```python
from build123d import *

# Parameters (mm, degrees)
BOSS_EXTRUDE1_DEPTH = 30
SKETCH2_R           = 2
CUT_EXTRUDE1_DEPTH  = 3
FILLET1_R           = 3


with BuildPart() as part:
    # Sketch1 → Boss-Extrude1 (new body)
    with BuildSketch(Plane(origin=(-298.953701388, 67.353578403, 0), x_dir=(1, 0, 0), z_dir=(0, 0, 1))):
        Polygon((318.453701388, -54.353578403), (318.453701388, -64.353578403), (313.453701388, -64.353578403), (313.453701388, -54.353578403), (310.453701388, -54.353578403), (310.453701388, -64.353578403), (298.953701388, -64.353578403), (298.953701388, -67.353578403), (332.953701388, -67.353578403), (332.953701388, -64.353578403), (321.453701388, -64.353578403), (321.453701388, -54.353578403), align=None)
    extrude(amount=BOSS_EXTRUDE1_DEPTH)

    # Sketch2 → Cut-Extrude1 (cut)
    with BuildSketch(Plane(origin=(0, 3, 0), x_dir=(1, 0, 0), z_dir=(0, 1, 0))):
        with Locations(Location((29, -6, 0), (0, 0, 270))):
            Circle(SKETCH2_R)
        with Locations(Location((29, -24, 0), (0, 0, 270))):
            Circle(SKETCH2_R)
    cut_extrude1 = extrude(amount=-CUT_EXTRUDE1_DEPTH, mode=Mode.SUBTRACT)

    # Mirror1: Cut-Extrude1 across plane
    add(cut_extrude1.mirror(Plane(origin=(17, 0, 0), x_dir=(0, 0, 1), z_dir=(1, 0, 0))), mode=Mode.SUBTRACT)

    # Fillet1
    fillet1_edges = [part.edges().sort_by_distance(p)[0] for p in [
        (11.5, 3, 15),
        (22.5, 3, 15),
    ]]
    fillet(fillet1_edges, radius=FILLET1_R)


solid = part.part
```
Part model, mm, in its own coordinate system. A direction names the side the tool comes from. Round coordinates to 2 decimals unless told otherwise and drop trailing zeros. Order: outer loops, then holes, each group sorted by start corner. A loop starts at its lowest first (then second) coordinate and runs counter-clockwise, first axis right, second up. Notation, with made-up numbers: M 54.25,89 L 95.25,89 A16 cw 95.25,99 Z; hole C 35.5,51 d1. An arc over 180 degrees is marked long. Answer in a Markdown table with one row per item. Add a question column.
Q1. Wall check: L1, parallel to Z at x = 5, y = 0.6; L2, parallel to X at y = 0.8, z = 24; L3, parallel to X at y = 2.25, z = 7.5. Give the ranges that are in metal, low to high. Write a range as from..to.
Q2. 3-axis set-ups, long thin cutter, end or side, ignore diameter. For faces 4 (the face through (6.2, 1.5, 22.4)), 5 (the face through (17, 2, 30)), 6 (the face through (19.5, 8, 15)), 7 (the face through (4, 3, 15)), 8 (the face through (30, 3, 15)): which of +Z, -Z, +X, -X, +Y, -Y reach the whole face in a straight line?
Q3. Mould opens along X. For faces 1 (the face through (6.2, 1.5, 4.4)), 2 (the face through (22.5, 9, 15)), 3 (the face through (0, 2, 15)) say: +X half, -X half, draft (parallel to the pull), parting line (faces both ways), or undercut.
Q4. Cut at B-B on y = 8.75. Give the cut face in (x, z).
Q5. Pin check, flat tips, straight feed: pin 1 (5 mm diameter, centred on x = 29, z = 6, fed in from +Y); pin 2 (3 mm diameter, centred on x = 5, z = 24, fed in from -Y); pin 3 (3.5 mm diameter, centred on y = 11, z = 22, fed in from +X); pin 4 (6 mm diameter, centred on x = 7.5, z = 24, fed in from +Y). Stop position of each tip, or through.
Q6. Cut at A-A on x = 5. Give the cut face in (y, z).
Q7. Cut at D-D on y = 1.75. Give the cut face in (x, z), and give its area (3 significant figures).
Q8. Cut at C-C on z = 6. Give the cut face in (x, y), and give its area (3 significant figures).
Established:
| question | item | result |
|---|---|---|
| 1 | L1 | z = 0..4, 8..22, 26..30 |
| 1 | L2 | x = 0..3, 7..27, 31..34 |
| 1 | L3 | x = 0..3.68, 6.32..27.68, 30.32..34 |
| 2 | face 4 | +Y, -Y |
| 2 | face 5 | +Z, +X, -X, +Y, -Y |
| 2 | face 6 | +Z, -Z, +Y |
| 2 | face 7 | +Z, -Z, -X, +Y |
| 2 | face 8 | +Z, -Z, +X, +Y |
| 3 | face 1 | undercut |
| 3 | face 2 | +X half |
| 3 | face 3 | -X half |
| 4 | outline | M 11.5,0 L 14.5,0 L 14.5,30 L 11.5,30 Z; M 19.5,0 L 22.5,0 L 22.5,30 L 19.5,30 Z |
| 5 | pin 1 | stops at y = 3 |
| 5 | pin 2 | passes through |
| 5 | pin 3 | stops at x = 22.5 |
| 5 | pin 4 | stops at y = 3.76 |
| 6 | outline | M 0,0 L 3,0 L 3,4 L 0,4 Z; M 0,8 L 3,8 L 3,22 L 0,22 Z; M 0,26 L 3,26 L 3,30 L 0,30 Z |
| 7 | outline | M 0,0 L 34,0 L 34,30 L 0,30 Z; hole C 5,6 d4; hole C 5,24 d4; hole C 29,6 d4; hole C 29,24 d4 |
| 7 | area | 970 mm2 |
| 8 | outline | M 0,0 L 3,0 L 3,3 L 0,3 Z; M 7,0 L 27,0 L 27,3 L 25.5,3 A3 cw 22.5,6 L 22.5,13 L 19.5,13 L 19.5,3 L 14.5,3 L 14.5,13 L 11.5,13 L 11.5,6 A3 cw 8.5,3 L 7,3 Z; M 31,0 L 34,0 L 34,3 L 31,3 Z |
| 8 | area | 142 mm2 |
